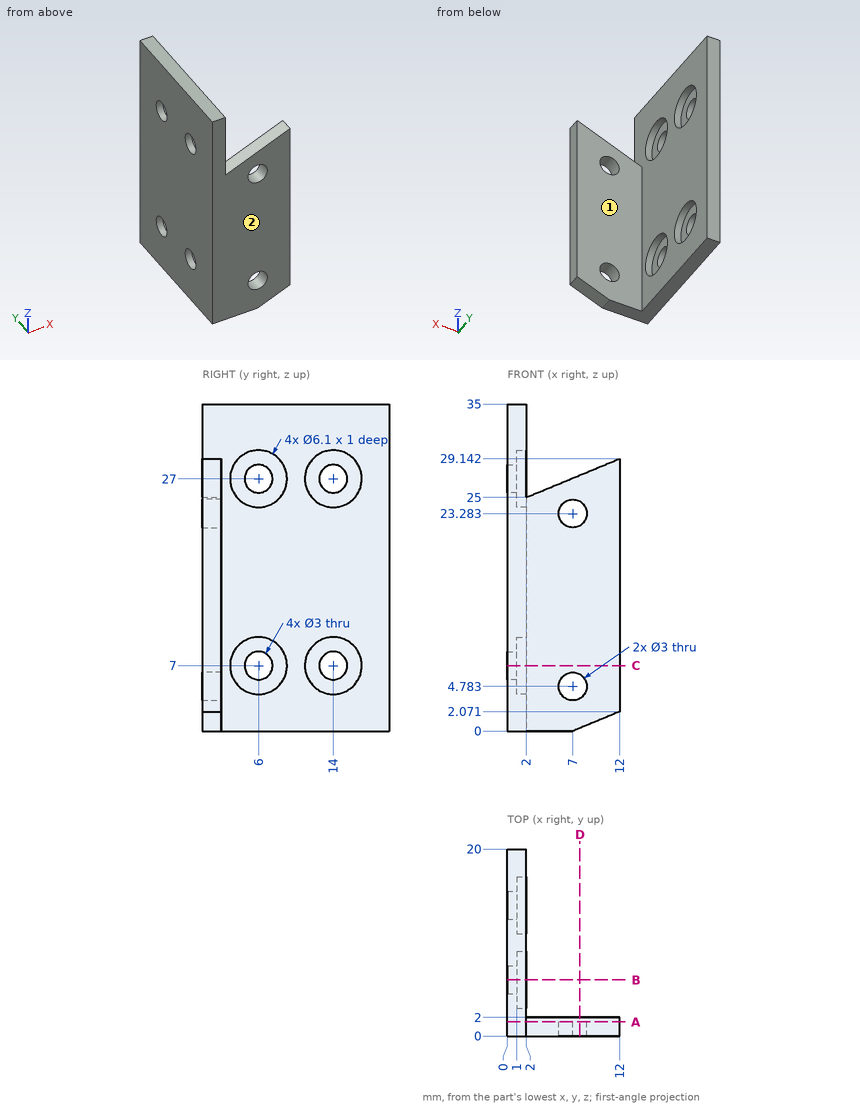
Input: dimensioned drawing with shaded views. Units: mm. Origin: part minimum x, y, z. A direction names the side the tool comes from. Coordinates: 2 decimals unless noted, no trailing zeros. Write each loop counter-clockwise with the first axis right and the second up, starting at its lowest first coordinate (ties: lowest second). Pieces come first, ordered by that corner, then holes. Notation, with made-up numbers: M 53,52 L 68,52 A26 ccw 68,81 Z; hole C 81,85.5 d9. An arc over 180 degrees is marked long. Use a Markdown table: item, result.
1) Section A-A, the plane y = 1.5. Output: boundary loops of the cut face in (x, z).
Conclusion:
| item | result |
|---|---|
| outline | M 0,0 L 7,0 L 12,2.07 L 12,29.14 L 2,25 L 2,35 L 0,35 Z; hole C 7,4.78 d3; hole C 7,23.28 d3 |
2) Section C-C, the plane z = 7. Output: boundary loops of the cut face in (x, y).
Conclusion:
| item | result |
|---|---|
| outline | M 0,0 L 12,0 L 12,2 L 2,2 L 2,2.95 L 1,2.95 L 1,4.5 L 0,4.5 Z; M 0,7.5 L 1,7.5 L 1,9.05 L 2,9.05 L 2,10.95 L 1,10.95 L 1,12.5 L 0,12.5 Z; M 0,15.5 L 1,15.5 L 1,17.05 L 2,17.05 L 2,20 L 0,20 Z |
3) Ray query, L1, parallel to Y at x = 1.4, z = 27; L2, parallel to Y at x = 0.7, z = 7; L3, parallel to Z at x = 0.5, y = 6.5 (1 decimal). Return the intervals inside material, ascending.
Conclusion:
| item | result |
|---|---|
| L1 | y = 0 to 2.95, 9.05 to 10.95, 17.05 to 20 |
| L2 | y = 0 to 4.5, 7.5 to 12.5, 15.5 to 20 |
| L3 | z = 0 to 5.6, 8.4 to 25.6, 28.4 to 35 |
4) Section B-B, the plane y = 6. Output: boundary loops of the cut face in (x, z), then the cut area to 3 significant figures.
Conclusion:
| item | result |
|---|---|
| outline | M 0,0 L 2,0 L 2,3.95 L 1,3.95 L 1,5.5 L 0,5.5 Z; M 0,8.5 L 1,8.5 L 1,10.05 L 2,10.05 L 2,23.95 L 1,23.95 L 1,25.5 L 0,25.5 Z; M 0,28.5 L 1,28.5 L 1,30.05 L 2,30.05 L 2,35 L 0,35 Z |
| area | 51.8 mm^2 |
5) Section D-D, the plane x = 7.75. Output: boundary loops of the cut face in (y, z).
Conclusion:
| item | result |
|---|---|
| outline | M 0,0.31 L 2,0.31 L 2,3.48 L 0,3.48 Z; M 0,6.08 L 2,6.08 L 2,21.98 L 0,21.98 Z; M 0,24.58 L 2,24.58 L 2,27.38 L 0,27.38 Z |
6) Reachability of the marked faces 1 and 2 from +Z, -Z, +X, -X, +Y, -Y: full face, straight path, thin tool, end or side. Return the list, or none.
Conclusion:
| item | result |
|---|---|
| face 1 | +Z, -Z, +X, +Y |
| face 2 | +Z, -Z, +X, -X, -Y |
7) First-contact query: pin 1 Ø4 at (x, z) = (7, 23.28) entering from +Y; pin 2 Ø5 at (y, z) = (15, 28) entering from +X; pin 3 Ø5 at (y, z) = (6, 27) entering from +X; pin 4 Ø2.5 at (x, z) = (7, 4.78) entering from -Y. Flat tips, straight axial feed; report the tip coordinate or a pass-through.
Conclusion:
| item | result |
|---|---|
| pin 1 | stops at y = 2 |
| pin 2 | stops at x = 2 |
| pin 3 | stops at x = 1 |
| pin 4 | passes through |
